Could you check a few things on this model? Use its own coordinates, in mm. Face numbers are marked on the shaded views. Give positions to 0.01 mm unless a question says otherwise; leave off trailing zeros. Loops run counter-clockwise (first coordinate to the right, second up) from the corner with the lowest first, then second, coordinate; pieces in that order, holes last. Notation, with made-up numbers: M 18.25,73 L 49.25,73 A13 ccw 49.25,91 Z; hole C 23,82 d10. An arc over 180 degrees is marked long. Use a Markdown table: item, result. Add a question column.
1) If I drill on line 1 along Y through (x, z) = (0, 1.1); line 2 along Y through (x, z) = (-0.75, 1.8); line 3 along X through (y, z) = (-19, 0.25), over which ranges is the centre line in solid material (lowest first)? Write a range as [from, to].
2) Will this pin go through, and if not, where does the flat tip stop? pin 1 Ø8.5 at (x, y) = (0, -20) entering from +Z.
3) Suppose I cut it at C-C on x = 0. List the corners of the cut face in (y, z) for me, and give its area (3 significant figures).
4) We'd pull the mould along Y, two halves only. Please class the marked faces 1, 2, 3 and 4: +Y half, -Y half, draft (parallel to the pull), parting line (faces both ways), or undercut.
5) Suppose I cut it at A-A on z = 1.25. List the corners of the cut face in (x, y) for me, and give its area (3 significant figures).
6) Suppose I cut it at B-B on y = 0. List the corners of the cut face in (x, z) for me, and give its area (3 significant figures).
7) Suppose I cut it at D-D on x = -8.25. List the corners of the cut face in (y, z) for me.
Autodesk Inventor part; units mm, degrees
ref_plane "YZ Plane" through (0, 0, 0) normal (1, 0, 0) x (0, 1, 0)
ref_plane "XZ Plane" through (0, 0, 0) normal (0, 1, 0) x (-1, 0, 0)
ref_plane "XY Plane" through (0, 0, 0) normal (0, 0, 1) x (1, 0, 0)
sketch "Sketch1" plane through (0, 0, 0) normal (0, 0, 1) x (1, 0, 0)
  line L0 (0, 0) -> (0, 20) construction
  line L1 (0, 0) -> (0, 20) construction
  line L2 (0, 20) -> (0, -20) construction
  line L3 (-10, 20) -> (-10, -20)
  line L4 (10, -20) -> (10, 20)
  arc A0 (10, 20) -> (-10, 20) centre (0, 20) ccw
  arc A1 (-10, -20) -> (10, -20) centre (0, -20) ccw
  circle A2 centre (0, 20) radius 2.6
  line L5 (0, 0) -> (10, 0) construction
  circle A3 centre (0, -20) radius 2.6
  circle A4 centre (0, 0) radius 2.5
  dimension "d15" = 20
  dimension "d16" = 20
  dimension "d17" = 40
  dimension "d18" = 10
  dimension "d19" = 5.2
  dimension "d20" = 5
extrude "Extrusion1" add sketch "Sketch1" along normal blind 3
properties part number "FingerSupport"
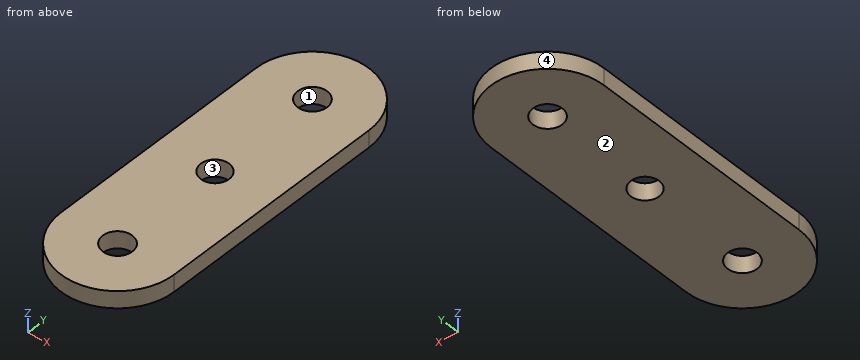
Answer block:
| question | item | result |
|---|---|---|
| 1 | line 1 | y = [-30, -22.6], [-17.4, -2.5], [2.5, 17.4], [22.6, 30] |
| 1 | line 2 | y = [-29.97, -22.49], [-17.51, -2.38], [2.38, 17.51], [22.49, 29.97] |
| 1 | line 3 | x = [-10, -2.4], [2.4, 10] |
| 2 | pin 1 | stops at z = 3 |
| 3 | outline | M -30,0 L -22.6,0 L -22.6,3 L -30,3 Z; M -17.4,0 L -2.5,0 L -2.5,3 L -17.4,3 Z; M 2.5,0 L 17.4,0 L 17.4,3 L 2.5,3 Z; M 22.6,0 L 30,0 L 30,3 L 22.6,3 Z |
| 3 | area | 134 mm^2 |
| 4 | face 1 | undercut |
| 4 | face 2 | draft |
| 4 | face 3 | undercut |
| 4 | face 4 | +Y half |
| 5 | outline | M -10,-20 A10 ccw 10,-20 L 10,20 A10 ccw -10,20 Z; hole C 0,-20 d5.2; hole C 0,20 d5.2; hole C 0,0 d5 |
| 5 | area | 1,050 mm^2 |
| 6 | outline | M -10,0 L -2.5,0 L -2.5,3 L -10,3 Z; M 2.5,0 L 10,0 L 10,3 L 2.5,3 Z |
| 6 | area | 45.0 mm^2 |
| 7 | outline | M -25.65,0 L 25.65,0 L 25.65,3 L -25.65,3 Z |
